Read the model definition and answer for the solid it produces. Units are mm, in the model's axes. A direction names the side the tool comes from. Coordinates: 2 decimals unless noted, no trailing zeros. Loops run counter-clockwise (first coordinate to the right, second up) from the corner with the lowest first, then second, coordinate; pieces in that order, holes last. Notation, with made-up numbers: (51.25, 44) -> (101.25, 44) arc R15 ccw to (101.25, 67) -> close; hole circle Ø6 at (38.5, 59). An arc over 180 degrees is marked (long way). Answer as CSV lines item,"result".
```python
from build123d import *

# Parameters (mm, degrees)
SKETCH_1_W                     = 39.3
SKETCH_1_H                     = 30
EXTRUDE_1_DEPTH                = 3
SKETCH_2_R                     = 1.525
EXTRUDE_2_DEPTH                = 3
SKETCH_4_R                     = 1.525
EXTRUDE_3_DEPTH                = 3
FILLET_1_R                     = 5
SKETCH_5_R                     = 1.525
CUT_EXTRUDE_1_DEPTH            = 30
SKETCH_6_R                     = 1.25
CUT_EXTRUDE_2_DEPTH            = 40
HOLE_WIZARD_M2_5_1_D           = 2.5
HOLE_WIZARD_M2_5_1_CSINK_D     = 5.4
HOLE_WIZARD_M2_5_1_CSINK_ANGLE = 90


with BuildPart() as part:
    # 草图1 → 凸台-拉伸1 (new body)
    with BuildSketch(Plane.XY):
        Rectangle(SKETCH_1_W, SKETCH_1_H)
    extrude(amount=EXTRUDE_1_DEPTH)

    # 草图2 → 凸台-拉伸2 (add)
    with BuildSketch(Plane.XY.offset(3)):
        with BuildLine():
            Line((-28.65, -7.5), (-19.65, -7.5))
            Line((-19.65, -7.5), (-19.65, -1.5))
            Line((-19.65, -1.5), (-28.65, -1.5))
            ThreePointArc((-28.65, -1.5), (-31.65, -4.5), (-28.65, -7.5))
        make_face()
        with Locations((-28.65, -4.5)):
            Circle(SKETCH_2_R, mode=Mode.SUBTRACT)
    extrude(amount=-EXTRUDE_2_DEPTH)

    # 草图4 → 凸台-拉伸3 (add)
    with BuildSketch(Plane.XY.offset(3)):
        with BuildLine():
            Line((28.65, 7.5), (19.65, 7.5))
            Line((19.65, 7.5), (19.65, 1.5))
            Line((19.65, 1.5), (28.65, 1.5))
            ThreePointArc((28.65, 1.5), (31.65, 4.5), (28.65, 7.5))
        make_face()
        with Locations((28.65, 4.5)):
            Circle(SKETCH_4_R, mode=Mode.SUBTRACT)
    extrude(amount=-EXTRUDE_3_DEPTH)

    # 圆角1
    fillet_1_edges = [part.edges().sort_by_distance(p)[0] for p in [
        (-19.65, -1.5, 1.5),
        (-19.65, -7.5, 1.5),
        (19.65, 1.5, 1.5),
        (19.65, 7.5, 1.5),
    ]]
    fillet(fillet_1_edges, radius=FILLET_1_R)

    # 草图5 → 切除-拉伸1 (cut)
    with BuildSketch(Plane.XY.offset(3)):
        with Locations((6, 10.5)):
            Circle(SKETCH_5_R)
        with Locations((-6, 10.5)):
            Circle(SKETCH_5_R)
        with Locations((-6, -10.5)):
            Circle(SKETCH_5_R)
        with Locations((6, -10.5)):
            Circle(SKETCH_5_R)
    extrude(amount=-CUT_EXTRUDE_1_DEPTH, mode=Mode.SUBTRACT)

    # 草图6 → 切除-拉伸2 (cut)
    with BuildSketch(Plane(origin=(0, 0, 0), x_dir=(-1, 0, 0), z_dir=(0, 0, -1))):
        with Locations((16.02146997, 9.25)):
            Circle(SKETCH_6_R)
        with Locations((-16.02146997, -9.25)):
            Circle(SKETCH_6_R)
        with Locations((16.02146997, -9.25)):
            Circle(SKETCH_6_R)
        with Locations((-16.02146997, 9.25)):
            Circle(SKETCH_6_R)
    extrude(amount=-CUT_EXTRUDE_2_DEPTH, mode=Mode.SUBTRACT)

    # M2.5 十字槽半沉头木螺钉的锥形沉头孔1 (through all)
    with Locations(Plane(origin=(0, 0, 0), x_dir=(-1, 0, 0), z_dir=(0, 0, -1))):
        with Locations((-16.02146997, 9.25), (-16.02146997, -9.25), (16.02146997, 9.25), (16.02146997, -9.25)):
            CounterSinkHole(HOLE_WIZARD_M2_5_1_D / 2, HOLE_WIZARD_M2_5_1_CSINK_D / 2, counter_sink_angle=HOLE_WIZARD_M2_5_1_CSINK_ANGLE)


solid = part.part
```
Q1. For a pull along X with two mould halves and no side action, classify faces 4 (the face through (16.18, 10.49, 2.21)), 5 (the face through (-29.8, -3.5, 1.5)), 6 (the face through (31.65, 4.43, 1.52)), 7 (the face through (0, 0, 0)) as pulls with the +X half, pulls with the -X half, needs draft (parallel to the pull), parting line crosses it, or undercut.
Results:
face 4,"undercut"
face 5,"undercut"
face 6,"pulls with the +X half"
face 7,"needs draft"
Q2. A cutting plane is placed at C-C, the plane y = -0.5. Write down the section's boundary in (x, z).
Results:
outline,"(-21.65, 0) -> (20.65, 0) -> (20.65, 3) -> (-21.65, 3) -> close"
Q3. A cutting plane is placed at D-D, the plane x = 21. Write down the section's boundary in (y, z), and give its area (3 significant figures).
Results:
outline,"(-0.08, 0) -> (9.08, 0) -> (9.08, 3) -> (-0.08, 3) -> close"
area,"27.5 mm²"
Q4. A cutting plane is placed at A-A, the plane y = -4.5. Write down the section's boundary in (x, z) (3 decimals).
Results:
outline,"(-31.65, 0) -> (-30.175, 0) -> (-30.175, 3) -> (-31.65, 3) -> close; (-27.125, 0) -> (19.65, 0) -> (19.65, 3) -> (-27.125, 3) -> close"
Q5. A cutting plane is placed at B-B, the plane x = -6. Write down the section's boundary in (y, z) (3 decimals).
Results:
outline,"(-15, 0) -> (-12.025, 0) -> (-12.025, 3) -> (-15, 3) -> close; (-8.975, 0) -> (8.975, 0) -> (8.975, 3) -> (-8.975, 3) -> close; (12.025, 0) -> (15, 0) -> (15, 3) -> (12.025, 3) -> close"
Q6. Given pin 1 Ø4 at (x, y) = (-6, -10.5) entering from +Z; pin 2 Ø1.5 at (x, z) = (27.5, 1.5) entering from -Y; pin 3 Ø1.5 at (x, y) = (16.02, -9.25) entering from -Z; pin 4 Ø0.9 at (x, z) = (27, 1) entering from +Y, each flat-ended and moving along its own axis, determine where each tip first touches the part or whether it passes through.
Results:
pin 1,"stops at z = 3"
pin 2,"stops at y = 1.5"
pin 3,"passes through"
pin 4,"stops at y = 7.5"
Q7. Find the intervals of material crossed by probe 1 along Y at (x, z) = (6, 1.6) (3 decimals); probe 2 along Y at (x, z) = (-28.65, 2.4) (3 decimals); probe 3 along Y at (x, z) = (-6.5, 0.75), in increasing order. Write a range as [from, to].
Results:
probe 1,"y = [-15, -12.025], [-8.975, 8.975], [12.025, 15]"
probe 2,"y = [-7.5, -6.025], [-2.975, -1.5]"
probe 3,"y = [-15, -11.94], [-9.06, 9.06], [11.94, 15]"
Q8. For faces 1 (the face through (-19.65, 9, 1)), 2 (the face through (27, 7.5, 2)), 3 (the face through (-19.65, -14, 1)), determine the directions among +Z, -Z, +X, -X, +Y, -Y from which every point of the face is accessible in a straight line to the end or side of a thin tool.
Results:
face 1,"+Z, -Z, -X, +Y"
face 2,"+Z, -Z, +X, +Y"
face 3,"+Z, -Z, -X, -Y"
